from build123d import *

# Parameters (mm, degrees)
F0_R     = 25.4
F1_DEPTH = 558.8
F2_R     = 14.224
F3_DEPTH = 37.846
F4_SIZE  = 0.762
F6_R     = 3.96875
F7_DEPTH = 6.35


with BuildPart() as f1:
    # F0 (on Front) → F1 (new body)
    with BuildSketch(Plane.XZ):
        Circle(F0_R)
    extrude(amount=F1_DEPTH)

    # F2 (on face) → F3 (join)
    with BuildSketch(Plane.XZ.offset(558.8)):
        Circle(F2_R)
    extrude(amount=F3_DEPTH)

    # F4
    f4_edges = [f1.edges().sort_by_distance(p)[0] for p in [
        (-14.224, -596.646, 0),
        (-25.4, -558.8, 0),
        (-25.4, 0, 0),
    ]]
    chamfer(f4_edges, length=F4_SIZE)

    # F6 (on offset) → F7 (cut)
    with BuildSketch(Plane.XY.offset(14.224)):
        with Locations((0, -577.596)):
            Circle(F6_R)
    extrude(amount=-F7_DEPTH, mode=Mode.SUBTRACT)


solid = f1.part
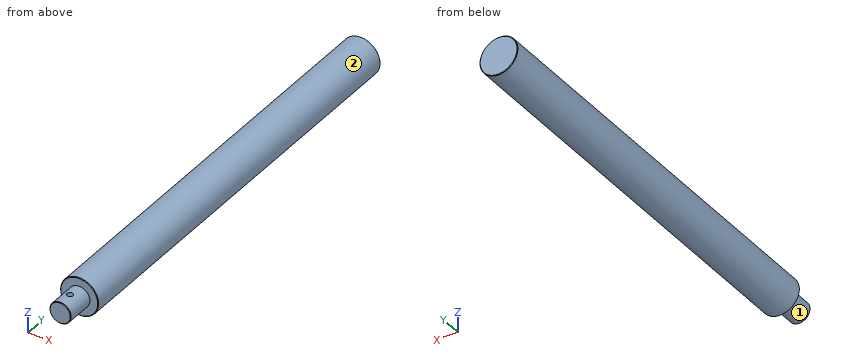
Read the model definition and answer for the solid it produces. Units are mm, in the model's axes. Face numbers are marked on the shaded views. A direction names the side the tool comes from. Coordinates: 2 decimals unless noted, no trailing zeros. Loops run counter-clockwise (first coordinate to the right, second up) from the corner with the lowest first, then second, coordinate; pieces in that order, holes last.
Q1. Which of the six approach directions +Z, -Z, +X, -X, +Y, -Y give full straight-line access (tool end or side, diameter ignored) to the marked faces 1 and 2?
Q2. Each of these flat-tipped pins is pushed along its axis until it touches: pin 1 Ø6 at (x, y) = (-9.5, -324) entering from -Z; pin 2 Ø5 at (x, z) = (-16, 5.5) entering from -Y; pin 3 Ø9 at (x, y) = (0, -577.596) entering from -Z. Where does it stop, or does it pass through?
Q3. The part is cut by section B-B on y = -93. Write down the section's boundary in (x, z), and give its area (3 significant figures).
Q4. Consider probe 1 along Y at (x, z) = (0, 11.25); probe 2 along Y at (x, z) = (7, -16.5); probe 3 along Z at (x, y) = (-2, -524). Determine where each line is inside the solid, lowest interval first.
Q5. The part is cut by section A-A on z = 0. Write down the section's boundary in (x, y), and give its area (3 significant figures).
Results below:
1. face 1: -Y
1. face 2: +Y, -Y
2. pin 1: stops at z = -24.55
2. pin 2: stops at y = -558.8
2. pin 3: stops at z = -14.22
3. outline: circle Ø50.8 at (0, 0)
3. area: 2,030 mm2
4. probe 1: y = -596.65 to -581.56, -573.63 to 0
4. probe 2: y = -558.8 to 0
4. probe 3: z = -25.32 to 25.32
5. outline: (-25.4, -558.04) - (-24.64, -558.8) - (-14.22, -558.8) - (-14.22, -595.88) - (-13.46, -596.65) - (13.46, -596.65) - (14.22, -595.88) - (14.22, -558.8) - (24.64, -558.8) - (25.4, -558.04) - (25.4, -0.76) - (24.64, 0) - (-24.64, 0) - (-25.4, -0.76) - close
5. area: 29,500 mm2
